For this review, take the finished solid that the model builds, in its own axes (mm). Face numbers are marked on the shaded views. A direction names the side the tool comes from. Round coordinates to 2 decimals unless told otherwise and drop trailing zeros. Order: outer loops, then holes, each group sorted by start corner. A loop starts at its lowest first (then second) coordinate and runs counter-clockwise, first axis right, second up. Notation, with made-up numbers: M 38.25,-18 L 43.25,-18 A20 cw 43.25,-5 Z; hole C 31.25,83.25 d7. An arc over 180 degrees is marked long. Write item = value, one per line. Start each with the question number.
from build123d import *

# Parameters (mm, degrees)
CROQUIS1_W              = 45
CROQUIS1_H              = 24.2
SALIENTE_EXTRUIR1_DEPTH = 10
CORTAR_EXTRUIR2_DEPTH   = 43
CROQUIS4_W              = 9.5
CROQUIS4_H              = 4.8
CORTAR_EXTRUIR3_DEPTH   = 48.659311787
CROQUIS5_W              = 12.2
CROQUIS5_H              = 1.6
CORTAR_EXTRUIR4_DEPTH   = 11
SALIENTE_EXTRUIR2_DEPTH = 2
SALIENTE_EXTRUIR3_DEPTH = 1.2
REDONDEO1_R             = 4
REDONDEO2_R             = 0.2


with BuildPart() as part:
    # Croquis1 → Saliente-Extruir1 (new body)
    with BuildSketch(Plane(origin=(0, 0, 0), x_dir=(1, 0, 0), z_dir=(0, 1, 0))):
        Rectangle(CROQUIS1_W, CROQUIS1_H)
    extrude(amount=SALIENTE_EXTRUIR1_DEPTH)

    # Croquis2 → Cortar-Extruir2 (cut)
    with BuildSketch(Plane(origin=(22.5, 0, 0), x_dir=(0, 0, -1), z_dir=(1, 0, 0))):
        Polygon((10.5, 1.6), (-10.5, 1.6), (-10.5, 3.6), (-9.7, 3.6), (-9.7, 8.4), (9.7, 8.4), (9.7, 3.6), (10.5, 3.6), align=None)
    extrude(amount=-CORTAR_EXTRUIR2_DEPTH, mode=Mode.SUBTRACT)

    # Croquis4 → Cortar-Extruir3 (cut, through all)
    with BuildSketch(Plane(origin=(22.5, 0, 0), x_dir=(0, 0, -1), z_dir=(1, 0, 0))):
        with Locations((2.25, 6)):
            Rectangle(CROQUIS4_W, CROQUIS4_H)
    extrude(amount=-CORTAR_EXTRUIR3_DEPTH, mode=Mode.SUBTRACT)

    # Croquis5 → Cortar-Extruir4 (cut)
    with BuildSketch(Plane(origin=(22.5, 0, 0), x_dir=(0, 0, -1), z_dir=(1, 0, 0))):
        with Locations((3.6, 9.2)):
            Rectangle(CROQUIS5_W, CROQUIS5_H)
    extrude(amount=-CORTAR_EXTRUIR4_DEPTH, mode=Mode.SUBTRACT)

    # Croquis6 → Saliente-Extruir2 (add)
    with BuildSketch(Plane(origin=(22.5, 0, 0), x_dir=(0, 0, -1), z_dir=(1, 0, 0))):
        Polygon((-2.5, 10), (-12.1, 10), (-12.1, 0), (-10.5, 0), (-10.5, 1.6), (-10.5, 3.6), (-9.7, 3.6), (-9.7, 8.4), (-2.5, 8.4), align=None)
        Polygon((12.1, 10), (9.7, 10), (9.7, 3.6), (10.5, 3.6), (10.5, 1.6), (10.5, 0), (12.1, 0), align=None)
    extrude(amount=SALIENTE_EXTRUIR2_DEPTH)

    # Croquis7 → Saliente-Extruir3 (add)
    with BuildSketch(Plane(origin=(24.5, 0, 0), x_dir=(0, 0, -1), z_dir=(1, 0, 0))):
        with BuildLine():
            Line((-10.5, 0), (10.5, 0))
            Line((10.5, 0), (10.5, 1.6))
            Line((10.5, 1.6), (6, 1.6))
            ThreePointArc((6, 1.6), (0, 2.6), (-6, 1.6))
            Line((-6, 1.6), (-10.5, 1.6))
            Line((-10.5, 1.6), (-10.5, 0))
        make_face()
    extrude(amount=-SALIENTE_EXTRUIR3_DEPTH)

    # Redondeo1
    redondeo1_edges = [part.edges().sort_by_distance(p)[0] for p in [
        (23.9, 1.6, 6),
        (23.9, 1.6, -6),
    ]]
    fillet(redondeo1_edges, radius=REDONDEO1_R)

    # Redondeo2
    redondeo2_edges = [part.edges().sort_by_distance(p)[0] for p in [
        (22.5, 0.8, -10.5),
        (23.3, 0.8, 10.5),
        (23.3, 0.8, -10.5),
        (22.5, 0.8, 10.5),
    ]]
    fillet(redondeo2_edges, radius=REDONDEO2_R)


solid = part.part
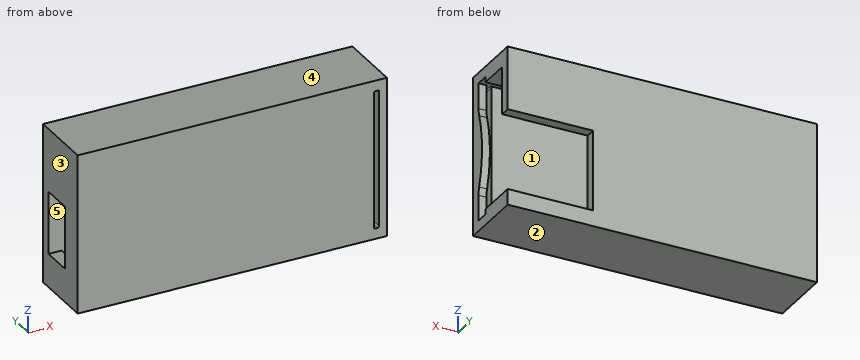
(1) For the marked faces 4 and 5, list the 3-axis set-ups (+Z, -Z, +X, -X, +Y, -Y) from which the entire face can be reached by the end or side of a thin tool; tool diameter is ignored.
(2) We need section A-A, the plane z = -7.5. Write out the cut boundary in (x, y), then the cut area to 3 significant figures.
(3) Insertion check: pin 1 (1.5 mm diameter, centred on x = 23.5, z = -8, fed in from +Y); pin 2 (3 mm diameter, centred on x = 18, z = 1.5, fed in from +Y). Each pin has a flat end and moves straight along its axis. Give the tip position at first contact, or say it passes through.
(4) We need section B-B, the plane x = -17.5. Write out the cut boundary in (y, z).
(5) For line 1 along Z through (x, y) = (-6, 3.5); line 2 along Y through (x, z) = (10, 6.25); line 3 along Z through (x, y) = (21, 4), list the stretches that pass through material, from the lowest coordinate up.
(6) We need section C-C, the plane y = 6.25. Write out the cut boundary in (x, z).
(7) Draft analysis for pull direction X (two halves, no side actions). For the marked faces 1, 2 and 3, state which applies: released by +X, released by -X, zero draft, split by the parting line, or undercut.
(8) We need section D-D, the plane y = 9.5. Write out the cut boundary in (x, z).
Values:
q1.face_4 = +Z, +X, -X, +Y, -Y
q1.face_5 = +X
q2.outline = M -22.5,0 L 22.5,0 L 22.5,1.6 L -20.5,1.6 L -20.5,8.4 L 11.5,8.4 L 11.5,10 L -22.5,10 Z; M 23.3,0 L 24.5,0 L 24.5,1.6 L 23.3,1.6 Z
q2.area = 142 mm²
q3.pin_1 = 1.6
q3.pin_2 = 10
q4.outline = M 0,-12.1 L 10,-12.1 L 10,12.1 L 0,12.1 Z; hole M 1.6,-10.5 L 3.6,-10.5 L 3.6,-9.7 L 8.4,-9.7 L 8.4,9.7 L 3.6,9.7 L 3.6,10.5 L 1.6,10.5 Z
q5.line_1 = -12.1 to -10.5, 10.5 to 12.1
q5.line_2 = 0 to 1.6, 8.4 to 10
q5.line_3 = -12.1 to -9.7, 9.7 to 12.1
q6.outline = M -22.5,-12.1 L 24.5,-12.1 L 24.5,-9.7 L -20.5,-9.7 L -20.5,-7 L -22.5,-7 Z; M -22.5,2.5 L -20.5,2.5 L -20.5,9.7 L 24.5,9.7 L 24.5,12.1 L -22.5,12.1 Z
q7.face_1 = undercut
q7.face_2 = zero draft
q7.face_3 = released by -X
q8.outline = M -22.5,-12.1 L 24.5,-12.1 L 24.5,-9.7 L 11.5,-9.7 L 11.5,2.5 L 24.5,2.5 L 24.5,12.1 L -22.5,12.1 Z
